Autodesk Fusion 360 part; units mm, degrees
sketch "Sketch1" plane through (0, 0, 0) normal (0, 0, 1) x (1, 0, 0)
  circle A0 centre (0, 0) radius 19 construction
  circle A1 centre (0, 0) radius 24 construction
  line L0 (-24, 0.0214) -> (24, 0.0214) construction
  line L1 (0, 0) -> (0, -50) construction
  line L2 (-25.5, 0) -> (-25.5, -50)
  line L3 (25.5, 0) -> (25.5, -50)
  line L4 (0, 0) -> (0, 24) construction
  line L5 (-25.5, 0) -> (-25.5, 0.25)
  line L6 (0, 24) -> (-1.75, 24)
  arc A2 (-1.75, 24) -> (-25.5, 0.25) centre (-1.75, 0.25) ccw
  arc A3 (25.5, 0.25) -> (1.75, 24) centre (1.75, 0.25) ccw
  line L7 (0, 24) -> (1.75, 24)
  line L8 (25.5, 0) -> (25.5, 0.25)
  dimension "d1" = 38
  dimension "d2" = 5
  dimension "d3" = 50
  dimension "d4" = 25.5
  dimension "d5" = 25.5
  dimension "d6" = 23.75
sketch "Sketch2" plane through (0, 0, 0) normal (1, 0, 0) x (0, 0, -1)
  circle A0 centre (0, 24) radius 5
  point P0 (0, 24)
  dimension "d7" = 10
sweep "Sweep1" add profiles "Sketch2" path "Sketch1" along L3 L8 A3 L7 L6 A2 L5 L2 section 1
chamfer "Chamfer1" distance 1.5 angle 45 2 edges at (-27.3081, -50, 4.6616) (23.6919, -50, 4.6616)
thread "Thread1"
thread "Thread2"
The listing builds one solid part. Answer for the finished solid, in the listing's coordinates (mm). A direction names the side the tool comes from. Round coordinates to 2 decimals unless told otherwise and drop trailing zeros. Write each loop counter-clockwise with the first axis right and the second up, starting at its lowest first coordinate (ties: lowest second). Pieces come first, ordered by that corner, then holes. Notation, with made-up numbers: (76, 59.25) - (96, 59.25) arc R5 ccw to (96, 68.25) - close; hole circle Ø8 at (74.25, -38.5). An arc over 180 degrees is marked (long way). Use one line per item in the form item = value. Start each with the question number.
Item 1: Find the intervals of material crossed by line 1 (X direction, y = -7.5, z = 0); line 2 (X direction, y = 1, z = -4.5); line 3 (Z direction, x = 16, y = 19), in increasing order. Write a range as [from, to].
Item 2: A tool of negligible diameter and unlimited length cuts with its end or side. For faces 1 (the cylindrical face through (0.02, 19.12, 1.08)), 2 (the flat face through (26, -50, 0)), 3 (the cylindrical face through (20.62, -24.47, 1.08)), from which of +Z, -Z, +X, -X, +Y, -Y can it reach the whole face along a straight path? Write none if from no direction.
Item 3: Flat-ended cylindrical pins translate along their axes: pin 1 Ø3 at (x, y) = (-16, 11.5) entering from +Z; pin 2 Ø1 at (x, z) = (-14, -1) entering from -Y; pin 3 Ø4 at (x, z) = (-6.5, 1.5) entering from +Y. Find the tip coordinate at first contact, or state that the pin passes through.
Item 4: A cutting plane is placed at A-A (z = 0). Write down the section's boundary in (x, y), plus the area to 3 significant figures.
Item 5: A cutting plane is placed at B-B (y = -36.5). Write down the section's boundary in (x, z).
The answers:
q1.line_1 = [-30.5, -20.5], [20.5, 30.5]
q1.line_2 = [-27.67, -23.31], [23.31, 27.67]
q1.line_3 = [-5, 5]
q2.face_1 = none
q2.face_2 = +Z, -Z, +X, -X, -Y
q2.face_3 = -Y
q3.pin_1 = 2.87
q3.pin_2 = 14.12
q3.pin_3 = 28.82
q4.outline = (-30.5, -48.5) - (-29, -50) - (-22, -50) - (-20.5, -48.5) - (-20.5, 0.25) arc R18.75 cw to (-1.75, 19) - (1.75, 19) arc R18.75 cw to (20.5, 0.25) - (20.5, -48.5) - (22, -50) - (29, -50) - (30.5, -48.5) - (30.5, 0.25) arc R28.75 ccw to (1.75, 29) - (-1.75, 29) arc R28.75 ccw to (-30.5, 0.25) - close
q4.area = 1,780 mm^2
q5.outline = circle Ø10 at (-25.5, 0); circle Ø10 at (25.5, 0)
